Autodesk Fusion 360 part; units mm, degrees
sketch "Sketch1" plane through (0, 0, 0) normal (0, 1, 0) x (1, 0, 0)
box "BoxPrimitive1" add length 6.5 width 9 height 3.6 placed x (0, 0, 1) y (1, 0, 0) z (0, 1, 0) at (0, 0, 0)
sketch "Sketch2" plane through (0, 0, 6.5) normal (0, 0, 1) x (1, 0, 0)
  line L0 (0, 3.6) -> (0, 0)
  line L1 (0, 0) -> (9, 0)
  line L2 (9, 0) -> (9, 3.6)
  line L3 (9, 3.6) -> (0, 3.6)
  line L4 (4.5, 3.6) -> (4.5, 0)
  line L5 (4.5, 1.8) -> (6.25, 1.8)
  line L6 (6.25, 1.8) -> (6.25, 1.05)
  line L7 (6.25, 1.05) -> (2.75, 1.05)
  line L8 (2.75, 1.05) -> (2.75, 2.55)
  line L9 (2.75, 2.55) -> (6.25, 2.55)
  line L10 (6.25, 2.55) -> (6.25, 1.8)
  line L11 (2.75, 2.55) -> (4.25, 2.55)
  line L12 (4.25, 2.55) -> (4.25, 1.05)
  dimension "d6" = 1.75
  dimension "d7" = 0.75
  dimension "d8" = 3.5
  dimension "d9" = 1.5
  dimension "d10" = 3.5
  dimension "d11" = 1.5
extrude "Extrude1" add sketch "Sketch2" along normal blind 2 contours L7 L8 L9 L11 L12
extrude "Extrude2" cut sketch "Sketch2" against normal blind 0.25 contours L4 L5 L9 L10 | L4 L7 L9 L12 | L4 L5 L6 L7

Autodesk Fusion 360 part; units mm, degrees
sketch "Sketch1" plane through (0, 0, 0) normal (0, 0, 1) x (1, 0, 0)
  line L0 (0, 0) -> (36, 0)
  line L1 (36, 0) -> (36, 29)
  line L2 (36, 29) -> (0, 29)
  line L3 (0, 29) -> (0, 0)
  dimension "d1" = 36
  dimension "d2" = 29
extrude "Extrude1" add sketch "Sketch1" along normal blind 4.75
fillet "Fillet1" radius 2 4 edges at (18, 0, 4.75) (18, 0, 0) (18, 29, 4.75) (18, 29, 0)
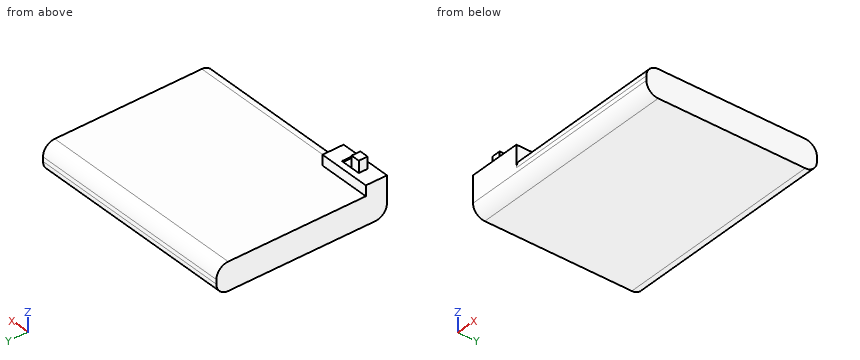
Part model, mm, in its own coordinate system. Round coordinates to 2 decimals unless told otherwise and drop trailing zeros. Loops run counter-clockwise (first coordinate to the right, second up) from the corner with the lowest first, then second, coordinate; pieces in that order, holes last. Notation, with made-up numbers: (50.5, 8) -> (66.5, 8) arc R22 cw to (66.5, 44) -> close; hole circle Ø11 at (33.25, 49.5). An arc over 180 degrees is marked (long way). Use a Markdown table: item, result.
1) Probe line 1 (Z direction, x = 25.5, y = 26.75); line 2 (Y direction, x = 3.5, z = 1); line 3 (Y direction, x = 25, z = 4). List the from-to ranges inside material, lowest first. Write a range as [from, to].
The answers:
| item | result |
|---|---|
| line 1 | z = [0, 4.75] |
| line 2 | y = [0.27, 28.73] |
| line 3 | y = [0.44, 28.56] |
2) Drop flat-ended pins along their axis: pin 1 Ø3 at (x, y) = (6, 1) entering from +Z; pin 2 Ø4 at (x, y) = (28.5, 19) entering from +Z; pin 3 Ø1.6 at (x, z) = (3.5, 7.5) entering from +Y. Give the stop position or say it passes through.
The answers:
| item | result |
|---|---|
| pin 1 | stops at z = 6.5 |
| pin 2 | stops at z = 4.75 |
| pin 3 | stops at y = 2.55 |
3) Cut at A-A, the plane x = 9.5. List the corners of the cut face in (y, z), and give its area (3 significant figures).
The answers:
| item | result |
|---|---|
| outline | (0, 2) arc R2 ccw to (2, 0) -> (27, 0) arc R2 ccw to (29, 2) -> (29, 2.75) arc R2 ccw to (27, 4.75) -> (2, 4.75) arc R2 ccw to (0, 2.75) -> close |
| area | 134 mm2 |
4) Cut at B-B, the plane y = 12.5. List the corners of the cut face in (x, z).
The answers:
| item | result |
|---|---|
| outline | (0, 0) -> (36, 0) -> (36, 4.75) -> (0, 4.75) -> close |
5) Cut at C-C, the plane z = 4. List the corners of the cut face in (x, y).
The answers:
| item | result |
|---|---|
| outline | (0, 0) -> (9, 0) -> (9, 0.44) -> (36, 0.44) -> (36, 28.56) -> (0, 28.56) -> close |
